Read the model definition and answer for the solid it produces. Units are mm, in the model's axes. Give positions to 0.01 mm unless a question says otherwise; leave off trailing zeros. One line per item, written item: value. Start each with the question number.
from build123d import *


with BuildPart() as part:
    # Esquisse1 → Base-Révolution (revolve)
    with BuildSketch(Plane(origin=(0, 0.557099225, 739.962502514), x_dir=(-1, 0, 0), z_dir=(0, -0.0007528747265126423, -0.9999997165897829)), mode=Mode.PRIVATE) as base_r_volution_sk:
        Polygon((-2199.400204284, 598.95640538), (-2198.900204284, 599.456870076), (-2198.908564931, 617.456867811), (-2199.408564931, 617.956403546), (-2205.408099158, 617.95361688), (-2206.908099158, 616.452222791), (-2206.902618614, 604.65292127), (-2205.402618773, 604.653617991), (-2205.400203367, 599.453386473), (-2204.900203367, 598.953850738), align=None)
    revolve(base_r_volution_sk.sketch.rotate(Axis((2192.899970054, 599.510903709, 739.511565204), (0.0004644803890833411, 0.9999996087187918, -0.0007528746453008684)), 270), axis=Axis((2192.899970054, 599.510903709, 739.511565204), (0.0004644803890833411, 0.9999996087187918, -0.0007528746453008684)))


solid = part.part
Item 1: Flat-ended cylindrical pins translate along their axes: pin 1 (3 mm diameter, centred on y = 614, z = 730, fed in from +X); pin 2 (6 mm diameter, centred on x = 2197.5, z = 735.5, fed in from +Y); pin 3 (3 mm diameter, centred on x = 2201.5, y = 608, fed in from -Z); pin 4 (10 mm diameter, centred on x = 2194, z = 731, fed in from -Y). Find the tip coordinate at first contact, or state that the pin passes through.
Item 2: Consider L1, parallel to X at y = 610.5, z = 739.5; L2, parallel to Y at x = 2185.5, z = 742; L3, parallel to X at y = 607.25, z = 744.5. Determine where each line is inside the solid, lowest interval first. Write a range as [from, to].
Item 3: Determine the mould class of faces 1 (the cylindrical face through (2180.485, 611.044, 745.963)), 2 (the cylindrical face through (2187.047, 609.144, 738.204)) for opening direction Z: pulls with the +Z half, pulls with the -Z half, needs draft (parallel to the pull), parting line crosses it, or undercut.
Computed values:
1. pin 1: x = 2204.4
1. pin 2: y = 618.51
1. pin 3: z = 727.44
1. pin 4: y = 599.51
2. L1: [2178.91, 2186.91], [2198.91, 2206.91]
2. L2: [599.52, 618.52]
2. L3: [2179.82, 2189.58], [2196.23, 2205.98]
3. face 1: parting line crosses it
3. face 2: undercut
